Build history of the part. All positions in model axes, mm. A direction names the side the tool comes from. Give positions to 0.01 mm unless a question says otherwise; leave off trailing zeros. Put each result on its own line as item: value.
from build123d import *

# Parameters (mm, degrees)
F0_W     = 23
F0_H     = 1
F0_W_2   = 1
F1_DEPTH = 3.75
F2_DEPTH = 2.6
F0_R     = 1
F0_R_2   = 8.5
F3_DEPTH = 1
F4_R     = 0.99999


# Not quite as in the source:
# - a fillet or chamfer is up to 0.001 mm smaller than in the source, because OpenCascade refuses the exact size


with BuildPart() as f1:
    # F0 (on Front) → F1 (new body)
    with BuildSketch(Plane.XZ):
        Polygon((-12.5, -13), (-12.5, -12), (-12.5, 12), (-12.5, 13), (-13.5, 13), (-13.5, -13), align=None)
        Polygon((12.5, 12), (12.5, -12), (12.5, -13), (13.5, -13), (13.5, 13), (12.5, 13), align=None)
        with Locations((0, -12.5)):
            Rectangle(F0_W, F0_H)
        with Locations((-12, -12.5)):
            Rectangle(F0_W_2, F0_H)
        with Locations((12, -12.5)):
            Rectangle(F0_W_2, F0_H)
    extrude(amount=F1_DEPTH)

    # F0 (on Front) → F2 (join)
    with BuildSketch(Plane.XZ):
        Polygon((-12.5, -12), (-11.5, -12), (-11.5, -10), (-11.5, 2.5), (-11.5, 12), (-12.5, 12), align=None)
        Polygon((11.5, -12), (12.5, -12), (12.5, 12), (11.5, 12), (11.5, 2.5), (11.5, -10), align=None)
    extrude(amount=F2_DEPTH)

    # F0 (on Front) → F3 (join)
    with BuildSketch(Plane.XZ):
        Polygon((-11.5, -12), (11.5, -12), (11.5, -10), (11.5, 2.5), (11.5, 12), (-11.5, 12), (-11.5, 2.5), (-11.5, -10), align=None)
        with BuildLine():
            ThreePointArc((-9.5, -10), (-10.5, -11), (-11.5, -10))
            ThreePointArc((-11.5, -10), (-10.5, -9), (-9.5, -10))
        make_face(mode=Mode.SUBTRACT)
        with Locations((10.5, -10)):
            Circle(F0_R, mode=Mode.SUBTRACT)
        with BuildLine():
            ThreePointArc((-9.5, 2.5), (-10.5, 1.5), (-11.5, 2.5))
            ThreePointArc((-11.5, 2.5), (-10.5, 3.5), (-9.5, 2.5))
        make_face(mode=Mode.SUBTRACT)
        Circle(F0_R_2, mode=Mode.SUBTRACT)
        with Locations((10.5, 2.5)):
            Circle(F0_R, mode=Mode.SUBTRACT)
        with Locations((0, 12.5)):
            Rectangle(F0_W, F0_H)
        Polygon((-12.5, -13), (-12.5, -12), (-12.5, 12), (-12.5, 13), (-13.5, 13), (-13.5, -13), align=None)
        Polygon((-12.5, -12), (-11.5, -12), (-11.5, -10), (-11.5, 2.5), (-11.5, 12), (-12.5, 12), align=None)
        with Locations((-12, 12.5)):
            Rectangle(F0_W_2, F0_H)
        with Locations((-12, -12.5)):
            Rectangle(F0_W_2, F0_H)
        with Locations((0, -12.5)):
            Rectangle(F0_W, F0_H)
        with Locations((12, -12.5)):
            Rectangle(F0_W_2, F0_H)
        Polygon((11.5, -12), (12.5, -12), (12.5, 12), (11.5, 12), (11.5, 2.5), (11.5, -10), align=None)
        Polygon((12.5, 12), (12.5, -12), (12.5, -13), (13.5, -13), (13.5, 13), (12.5, 13), align=None)
        with Locations((12, 12.5)):
            Rectangle(F0_W_2, F0_H)
    extrude(amount=-F3_DEPTH)

    # F4 (radius 1 in the source; OpenCascade refuses exactly that, so slightly less here)
    f4_edges = [f1.edges().sort_by_distance(p)[0] for p in [
        (-13.5, -3.75, 0),
        (13.5, -3.75, 0),
        (0, -3.75, -13),
        (-13.5, -1.375, 13),
        (13.5, -1.375, 13),
        (-13, -3.75, 13),
        (13, -3.75, 13),
        (11.5, -1.3, 12),
        (-11.5, -1.3, 12),
        (-8.5, 0, 0),
    ]]
    fillet(f4_edges, radius=F4_R)


solid = f1.part
1) Pull direction X, two halves, no side cores. Call faces 1 (the flat face through (-12.5, -3, 1)), 2 (the cylindrical face through (13.199, -0.849, 12.715)), 3 (the flat face through (0, 1, 9)): released by +X, released by -X, zero draft, split by the parting line, or undercut.
Filled sheet:
face 1: undercut
face 2: released by +X
face 3: zero draft
2) Tool access for faces 4 (the cylindrical face through (-13.215, -0.849, 12.699)), 5 (the cylindrical face through (11.785, -1.318, 11.699)): list every direction of +Z, -Z, +X, -X, +Y, -Y with a clear straight run to the whole face (end or side of a thin tool).
Filled sheet:
face 4: +Z, -X, +Y, -Y
face 5: +Z, -Y
3) Wall check: L1, parallel to Z at x = -10.5, y = 0.4; L2, parallel to X at y = -2.2, z = -7.75; L3, parallel to Z at x = -10.5, y = -1.6. Give the ranges that are in metal, low to high.
Filled sheet:
L1: -13 to -11, -9 to 1.5, 3.5 to 13
L2: -13.5 to -11.5, 11.5 to 13.5
L3: -13 to -12
4) Slice it at A-A (x = 10.5). Give the number of separate pieces and of enclosed holes in the cut face, plus the area to 3 significant figures.
Filled sheet:
separate pieces: 3
enclosed holes: 0
area: 25.5 mm2
5) Pin check, flat tips, straight feed: pin 1 (1.5 mm diameter, centred on x = 1.5, y = -3, fed in from +Z); pin 2 (3 mm diameter, centred on x = 10.5, z = -10, fed in from -Y); pin 3 (13.5 mm diameter, centred on x = 0, z = 0, fed in from -Y); pin 4 (8 mm diameter, centred on x = -0.5, z = -7.5, fed in from -Y). Stop position of each tip, or through.
Filled sheet:
pin 1: z = -12
pin 2: y = -2.6
pin 3: through
pin 4: y = 0
